from build123d import *

# Parameters (mm, degrees)
SKETCH1_R           = 29.65
BOSS_EXTRUDE1_DEPTH = 28.5
CHAMFER1_SIZE       = 10
FILLET1_R           = 5
SKETCH2_R           = 1.5
SKETCH2_R_2         = 2.429720262
CUT_EXTRUDE1_DEPTH  = 9.5
SKETCH3_R           = 1.5
CUT_EXTRUDE2_DEPTH  = 9.5


with BuildPart() as part:
    # Sketch1 → Boss-Extrude1 (new body)
    with BuildSketch(Plane.XY):
        with Locations((-37.247490996, 0)):
            Circle(SKETCH1_R)
    extrude(amount=BOSS_EXTRUDE1_DEPTH)

    # Chamfer1
    chamfer1_edges = [part.edges().sort_by_distance(p)[0] for p in [
        (-66.897490996, 0, 28.5),
    ]]
    chamfer(chamfer1_edges, length=CHAMFER1_SIZE)

    # Fillet1
    fillet1_edges = [part.edges().sort_by_distance(p)[0] for p in [
        (-66.897490996, 0, 0),
    ]]
    fillet(fillet1_edges, radius=FILLET1_R)

    # Sketch2 → Cut-Extrude1 (cut)
    with BuildSketch(Plane.XY.offset(28.5)):
        with Locations((-37.247490996, 6)):
            Circle(SKETCH2_R)
        with Locations((-43.247490996, 0)):
            Circle(SKETCH2_R)
        with Locations((-37.247490996, -6)):
            Circle(SKETCH2_R)
        with Locations((-31.247490996, 0)):
            Circle(SKETCH2_R)
        with Locations((-37.247490996, 0)):
            Circle(SKETCH2_R_2)
    extrude(amount=-CUT_EXTRUDE1_DEPTH, mode=Mode.SUBTRACT)

    # Sketch3 → Cut-Extrude2 (cut)
    with BuildSketch(Plane(origin=(0, 0, 0), x_dir=(-1, 0, 0), z_dir=(0, 0, -1))):
        with Locations((37.247490996, 12.5)):
            Circle(SKETCH3_R)
        with Locations((49.747490996, 0)):
            Circle(SKETCH3_R)
        with Locations((24.761374027, 0.588967782)):
            Circle(SKETCH3_R)
        with Locations((37.247490996, -12.5)):
            Circle(SKETCH3_R)
    extrude(amount=-CUT_EXTRUDE2_DEPTH, mode=Mode.SUBTRACT)


solid = part.part
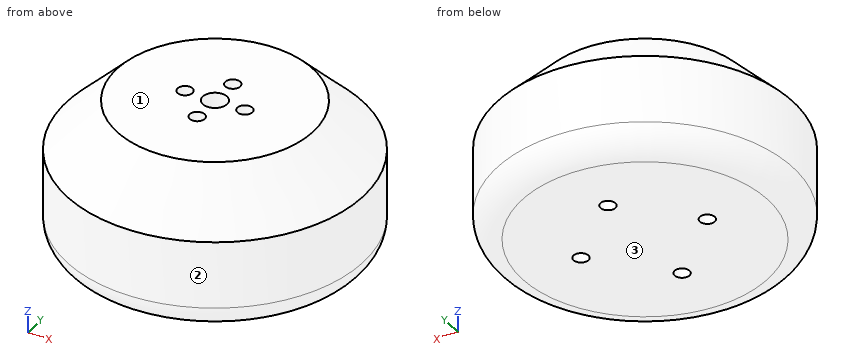
Design review of the part built by this model. Coordinates are the model's own, in mm. Face numbers are marked on the shaded views. Round coordinates to 2 decimals unless told otherwise and drop trailing zeros. Order: outer loops, then holes, each group sorted by start corner. A loop starts at its lowest first (then second) coordinate and runs counter-clockwise, first axis right, second up.
1) Draft analysis for pull direction Z (two halves, no side actions). For the marked faces 1, 2 and 3, state which applies: released by +Z, released by -Z, zero draft, split by the parting line, or undercut.
The answers:
face 1: released by +Z
face 2: zero draft
face 3: released by -Z
2) Consider section B-B (z = 17.5). State the section outline as (x, y) points.
The answers:
outline: circle Ø59.3 at (-37.25, 0)
3) For L1, parallel to X at y = 0.5, z = 19.75; L2, parallel to Y at x = -24, z = 3; L3, parallel to Z at x = -43, y = -21, list the stretches that pass through material, from the lowest coordinate up.
The answers:
L1: x = -65.64 to -44.66, -41.83 to -39.63, -34.87 to -32.66, -29.83 to -8.85
L2: y = -26.06 to -0.7, 1.88 to 26.06
L3: z = 0 to 26.38
4) Clearance check with flat-ended pins moving along their axes: pin 1 Ø1.5 at (x, y) = (-43.5, 0) entering from +Z; pin 2 Ø2.5 at (x, y) = (-37.25, -12.5) entering from -Z; pin 3 Ø3 at (y, z) = (7.5, 17) entering from -X. State where each tip first meets the part, or that it passes through.
The answers:
pin 1: stops at z = 19
pin 2: stops at z = 9.5
pin 3: stops at x = -66.28
5) Consider section A-A (z = 27.25). State the section outline as (x, y) points.
The answers:
outline: circle Ø41.8 at (-37.25, 0); hole circle Ø3 at (-43.25, 0); hole circle Ø4.86 at (-37.25, 0); hole circle Ø3 at (-37.25, -6); hole circle Ø3 at (-37.25, 6); hole circle Ø3 at (-31.25, 0)
